Geometry check sheet. Reference: the model listing, model coordinates, mm. A direction names the side the tool comes from. Coordinates: 2 decimals unless noted, no trailing zeros. Order: outer loops, then holes, each group sorted by start corner. A loop starts at its lowest first (then second) coordinate and runs counter-clockwise, first axis right, second up. Notation, with made-up numbers: (57, 73.5) - (68, 73.5) arc R20 ccw to (68, 80.5) - close; hole circle Ø4 at (-20.75, 79). An arc over 180 degrees is marked (long way). Use CSV: the item, a comma, the result in double quotes. Start each with the question number.
1) Draft check along X on faces 3 (the flat face through (23, -18, 3)), 4 (the flat face through (-37.094, -10, 3)), 5 (the flat face through (0.34, -31.88, 2.96)). Enter one of: released by +X, released by -X, zero draft, split by the parting line, or undercut.
2) Tool access check on faces 1 (the flat face through (-18, 0, 3)), 2 (the cylindrical face through (-6.36, -23.64, 2.96)). Record the directions out of +Z, -Z, +X, -X, +Y, -Y that give a thin tool (end or side, any length) a straight path to the whole face; none if there is none.
3) Depth check by flat-ended pin: P1, Ø2, axis at x = -25.5, z = 3.5, coming from the -Y side; P2, Ø3, axis at x = 20.5, z = 2.5, coming from the +Y side; P3, Ø0.7, axis at y = -41.5, z = 1.5, coming from the -X side. Enter the tip coordinate at first touch or a pass-through.
4) Sectioned sample at C-C, the plane x = -26. Record the cut outline in (y, z).
5) Thickness scan on probe 1 along Y at (x, z) = (19.5, 5.75); probe 2 along Y at (x, z) = (-18, 3); probe 3 along Y at (x, z) = (22.5, 0.75). Record the ranges inside material, lowest first. Write a range as [from, to].
6) Sectioned sample at D-D, the plane z = 2.25. Count the separate pieces of the cut face and the enclosed holes in it, and give its area (3 significant figures).
7) Sectioned sample at B-B, the plane y = -25. Record the cut outline in (x, z), and give its area (3 significant figures).
8) Sectioned sample at A-A, the plane y = -31. Record the cut outline in (x, z), and give its area (3 significant figures).
from build123d import *

# Parameters (mm, degrees)
SKETCH_1_R      = 2.5
SKETCH_1_R_2    = 1.25
EXTRUDE_1_DEPTH = 6
FILLET_1_R      = 5
FILLET_2_R      = 1


with BuildPart() as part:
    # 草图1 → 凸台-拉伸1 (new body)
    with BuildSketch(Plane.XY):
        with BuildLine():
            Line((1.500025947, -1.999165895), (12.605850611, -16.800500463))
            ThreePointArc((12.605850611, -16.800500463), (13.664114192, -17.683421453), (15.005475182, -18))
            Line((15.005475182, -18), (30.306366751, -18))
            Line((30.306366751, -18), (30.306366751, -32.6148543))
            Line((30.306366751, -32.6148543), (30.306366751, -42))
            Line((30.306366751, -42), (10.306366751, -42))
            Line((10.306366751, -42), (10.306366751, -41.12210437))
            Line((10.306366751, -41.12210437), (-20.930018343, -19.75))
            Line((-20.930018343, -19.75), (-32.093633249, -19.75))
            ThreePointArc((-32.093633249, -19.75), (-35.629167155, -18.285533906), (-37.093633249, -14.75))
            Line((-37.093633249, -14.75), (-37.093633249, -5))
            ThreePointArc((-37.093633249, -5), (-35.629167155, -1.464466094), (-32.093633249, 0))
            Line((-32.093633249, 0), (-2.499348338, 0))
            ThreePointArc((-2.499348338, 0), (-0.263746688, -0.527630912), (1.500025947, -1.999165895))
        make_face()
        with Locations((20.306366751, -36)):
            Circle(SKETCH_1_R, mode=Mode.SUBTRACT)
        with Locations((20.306366751, -24)):
            Circle(SKETCH_1_R, mode=Mode.SUBTRACT)
        with Locations((-29.093633249, -4.875)):
            Circle(SKETCH_1_R_2, mode=Mode.SUBTRACT)
        with Locations((-29.093633249, -14.875)):
            Circle(SKETCH_1_R_2, mode=Mode.SUBTRACT)
        with BuildLine():
            Line((9.305741036, -32.39670638), (1.316615651, -21.749165895))
            ThreePointArc((1.316615651, -21.749165895), (-0.447156984, -20.277630912), (-2.682758634, -19.75))
            Line((-2.682758634, -19.75), (-17.388195941, -19.75))
            Line((-17.388195941, -19.75), (10.306366751, -38.698770243))
            Line((10.306366751, -38.698770243), (10.306366751, -35.397540485))
            ThreePointArc((10.306366751, -35.397540485), (10.049618348, -33.815907061), (9.305741036, -32.39670638))
        make_face(mode=Mode.SUBTRACT)
    extrude(amount=EXTRUDE_1_DEPTH)

    # 圆角1
    # the kernel refuses this fillet: 5 mm, written as the material it adds along each edge
    with BuildSketch(Plane(origin=(10.306366751, -38.698770243, 0), x_dir=(0, 1, 0), z_dir=(0, 0, 1))) as fillet_1_piece_1:
        with BuildLine():
            CenterArc((7.693275838, 2.389546239), FILLET_1_R, 145.619854071, 62.929086432)
            Line((3.566729735, 5.2129515), (3.484198813, 5.269419605))
            Line((3.484198813, 5.269419605), (-0.082530922, 0.056468105))
            Line((-0.082530922, 0.056468105), (0, -0.1))
            ThreePointArc((0, -0.1), (1.650614879, -0.1), (3.213388836, -0.047790925))
            Line((3.213388836, -0.047790925), (3.301229757, 0))
        make_face()
    extrude(amount=6)
    with BuildSketch(Plane(origin=(-17.388195941, -19.75, 0), x_dir=(0.8253092204879542, -0.5646810520794596, 0), z_dir=(0, 0, 1))) as fillet_1_piece_2:
        with BuildLine():
            CenterArc((15.8894472, 5), FILLET_1_R, 138.640890522, 131.359109478)
            Line((12.136533001, 8.30388181), (12.061474717, 8.369959446))
            ThreePointArc((12.061474717, 8.369959446), (6.011798395, 4.234471827), (-0.056468105, 0.082530922))
            Line((-0.056468105, 0.082530922), (0, -0.1))
            Line((0, -0.1), (15.8894472, -0.1))
            Line((15.8894472, -0.1), (15.8894472, 0))
        make_face()
    extrude(amount=6)

    # 圆角2
    fillet_2_edges = [part.edges().sort_by_distance(p)[0] for p in [
        (10.306366751, -35.397540485, 3),
    ]]
    fillet(fillet_2_edges, radius=FILLET_2_R)


solid = part.part
Evaluation:
1,face 3,"zero draft"
1,face 4,"released by -X"
1,face 5,"undercut"
2,face 1,"+Z, -Z, +X, -X, +Y"
2,face 2,"+Z, -Z"
3,P1,"y = -19.75"
3,P2,"y = -18"
3,P3,"x = 10.31"
4,outline,"(-19.75, 0) - (0, 0) - (0, 6) - (-19.75, 6) - close"
5,probe 1,"[-42, -38.37], [-33.63, -26.37], [-21.63, -18]"
5,probe 2,"[-21.75, 0]"
5,probe 3,"[-42, -37.2], [-34.8, -25.2], [-22.8, -18]"
6,separate pieces,"1"
6,enclosed holes,"5"
6,area,"1,490 mm²"
7,outline,"(-13.26, 0) - (-6.43, 0) - (-6.43, 6) - (-13.26, 6) - close; (3.76, 0) - (18.02, 0) - (18.02, 6) - (3.76, 6) - close; (22.6, 0) - (30.31, 0) - (30.31, 6) - (22.6, 6) - close"
7,area,"173 mm²"
8,outline,"(-4.49, 0) - (-0.95, 0) - (-0.95, 6) - (-4.49, 6) - close; (8.26, 0) - (30.31, 0) - (30.31, 6) - (8.26, 6) - close"
8,area,"154 mm²"
